Could you check a few things on this drawing? It's one solid part, dimensions in mm from its lowest x, y, z. A direction names the side the tool comes from. Give positions to 0.01 mm unless a question says otherwise; leave off trailing zeros. Loops run counter-clockwise (first coordinate to the right, second up) from the corner with the lowest first, then second, coordinate; pieces in that order, holes last. Notation, with made-up numbers: (57.25, 64) -> (69.25, 64) arc R19 ccw to (69.25, 73) -> close; hole circle Ø6 at (-37, 25.25). An arc over 180 degrees is marked (long way). One line per question, with ' | ' between items.
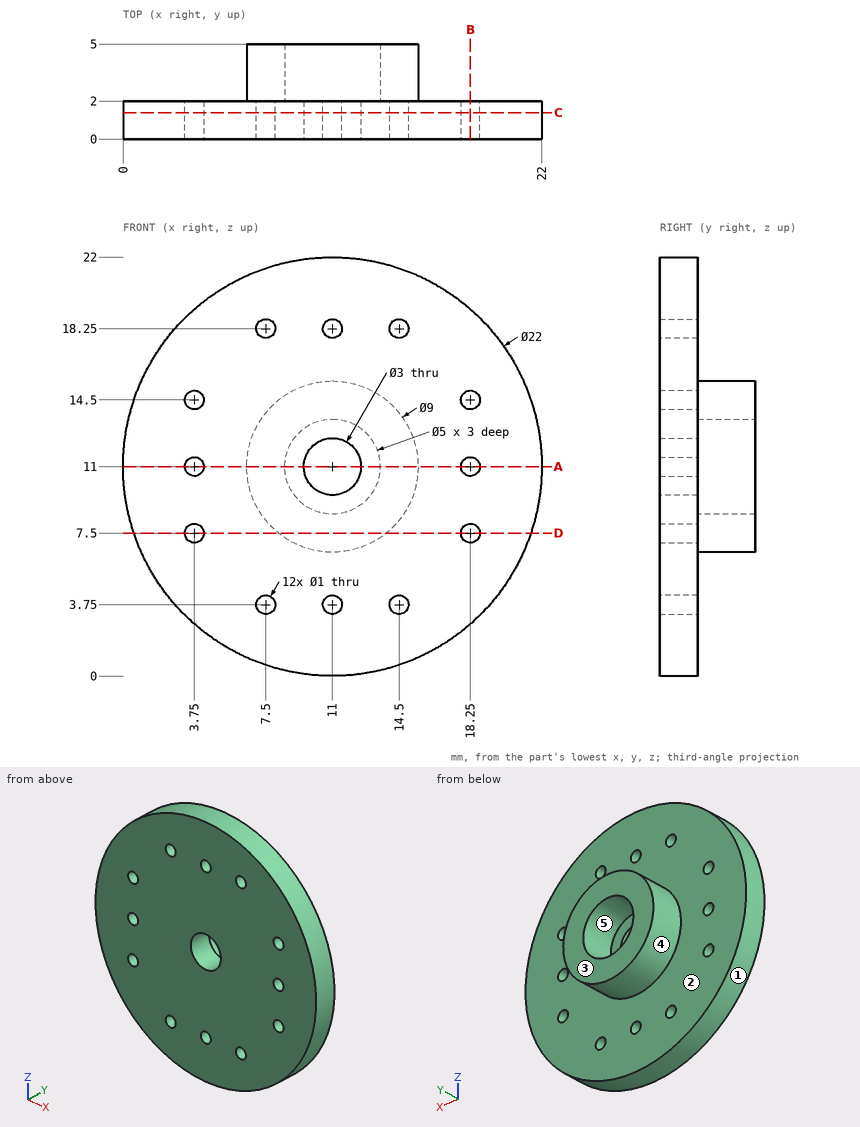
Q1. If we section it at A-A (z = 11): Write out the boundary of the cut face in (x, y).
Entries:
outline: (0, 0) -> (3.25, 0) -> (3.25, 2) -> (0, 2) -> close; (4.25, 0) -> (9.5, 0) -> (9.5, 2) -> (8.5, 2) -> (8.5, 5) -> (6.5, 5) -> (6.5, 2) -> (4.25, 2) -> close; (12.5, 0) -> (17.75, 0) -> (17.75, 2) -> (15.5, 2) -> (15.5, 5) -> (13.5, 5) -> (13.5, 2) -> (12.5, 2) -> close; (18.75, 0) -> (22, 0) -> (22, 2) -> (18.75, 2) -> close
Q2. For pin 1 Ø3 at (x, z) = (19, 17.5) entering from -Y; pin 2 Ø1.5 at (x, z) = (11.5, 10) entering from +Y; pin 3 Ø1.5 at (x, y) = (8, 1) entering from +Z; pin 4 Ø1 at (y, z) = (2, 18.5) entering from -X, each with a flat end and sliding along its axis, tell me the tip position at first contact or that it passes through.
Entries:
pin 1: y = 0 | pin 2: y = 2 | pin 3: z = 21.77 | pin 4: x = 2.51
Q3. If we section it at D-D (z = 7.5): Write out the boundary of the cut face in (x, y), plus the area to 3 significant figures.
Entries:
outline: (0.57, 0) -> (3.25, 0) -> (3.25, 2) -> (0.57, 2) -> close; (4.25, 0) -> (17.75, 0) -> (17.75, 2) -> (13.83, 2) -> (13.83, 5) -> (8.17, 5) -> (8.17, 2) -> (4.25, 2) -> close; (18.75, 0) -> (21.43, 0) -> (21.43, 2) -> (18.75, 2) -> close | area: 54.7 mm²
Q4. On a 3-axis mill with a long thin cutter (end or side, diameter ignored), from which of +Z, -Z, +X, -X, +Y, -Y can I reach the whole of each face in a straight line? I mean the marked faces 1 and 2. Say none if no direction works.
Entries:
face 1: +Y, -Y | face 2: +Y
Q5. If we section it at B-B (x = 18.25): Write out the boundary of the cut face in (y, z).
Entries:
outline: (0, 2.73) -> (2, 2.73) -> (2, 7) -> (0, 7) -> close; (0, 8) -> (2, 8) -> (2, 10.5) -> (0, 10.5) -> close; (0, 11.5) -> (2, 11.5) -> (2, 14) -> (0, 14) -> close; (0, 15) -> (2, 15) -> (2, 19.27) -> (0, 19.27) -> close
Q6. If I drill on probe 1 along X at (y, z) = (2.4, 11); probe 2 along X at (y, z) = (1.15, 18.25), over which ranges is the centre line in solid material (lowest first)? Write a range as from..to.
Entries:
probe 1: 6.5..8.5, 13.5..15.5 | probe 2: 2.73..7, 8..10.5, 11.5..14, 15..19.27
Q7. If we section it at C-C (y = 1.4): State how many separate pieces and enclosed holes the cut face has, plus the area to 3 significant figures.
Entries:
separate pieces: 1 | enclosed holes: 13 | area: 364 mm²
Q8. If we mould it in two halves opening along Z, with no side actions, what happens to the marked faces 3, 4 and 5? For each: pulls with the +Z half, pulls with the -Z half, needs draft (parallel to the pull), parting line crosses it, or undercut.
Entries:
face 3: needs draft | face 4: parting line crosses it | face 5: undercut
